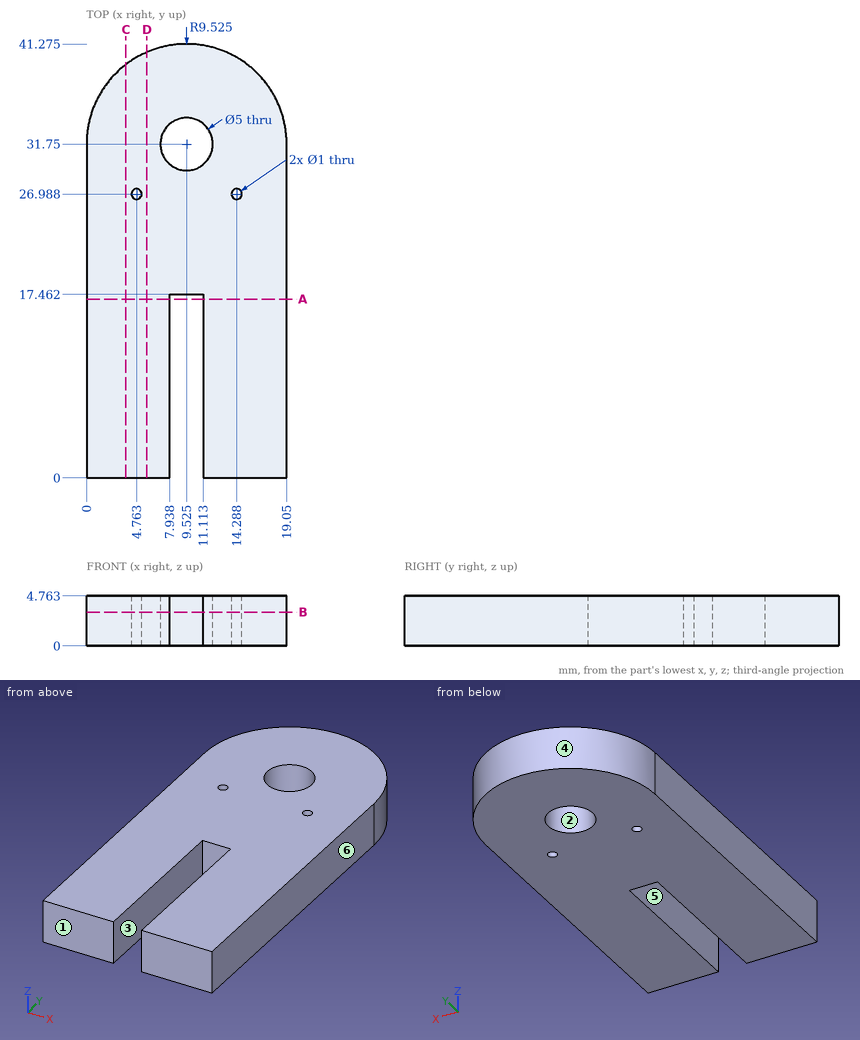
Print and shaded views of the part. All mm, measured from the part's lowest x, y and z. A direction names the side the tool comes from. Give positions to 0.01 mm unless a question says otherwise; leave off trailing zeros. Loops run counter-clockwise (first coordinate to the right, second up) from the corner with the lowest first, then second, coordinate; pieces in that order, holes last.
1) Pull direction X, two halves, no side cores. Call the marked faces 1, 2, 3 and 4: +X half, -X half, draft (parallel to the pull), parting line (faces both ways), or undercut.
2) Saw through at B-B (z = 3.2). Count the separate pieces of the cut face and the enclosed holes in it, plus the area to 3 significant figures.
3) Tool access for the marked faces 5 and 6: list every direction of +Z, -Z, +X, -X, +Y, -Y with a clear straight run to the whole face (end or side of a thin tool).
4) Flat gauge pins, fed straight in: pin 1 Ø8 at (x, y) = (7, 18.5) entering from -Z; pin 2 Ø1 at (x, z) = (9, 2.5) entering from -Y. Where does each tip first touch, or does it go through?
5) Saw through at D-D (x = 5.75). Write the cut outline in (y, z) (1 decimal), plus the area to 3 significant figures.
6) Saw through at A-A (y = 17). Write the cut outline in (x, z).
7) Wall check: line 1 (X direction, y = 10.5, z = 1.6); line 2 (X direction, y = 30, z = 4.2); line 3 (Y direction, x = 7.5, z = 0.2) (1 decimal). Give the ranges that are in metal, low to high.
8) Saw through at C-C (x = 3.75). Write the cut outline in (y, z) (1 decimal).
Answer block:
1. face 1: draft
1. face 2: undercut
1. face 3: undercut
1. face 4: parting line
2. separate pieces: 1
2. enclosed holes: 3
2. area: 671 mm2
3. face 5: +Z, -Z, -Y
3. face 6: +Z, -Z, +X, +Y, -Y
4. pin 1: stops at z = 0
4. pin 2: stops at y = 17.46
5. outline: (0, 0) - (40.5, 0) - (40.5, 4.8) - (0, 4.8) - close
5. area: 193 mm2
6. outline: (0, 0) - (7.94, 0) - (7.94, 4.76) - (0, 4.76) - close; (11.11, 0) - (19.05, 0) - (19.05, 4.76) - (11.11, 4.76) - close
7. line 1: x = 0 to 7.94, 11.11 to 19.05
7. line 2: x = 0 to 7.74, 11.31 to 19.05
7. line 3: y = 0 to 30.3, 33.2 to 41.1
8. outline: (0, 0) - (39.3, 0) - (39.3, 4.8) - (0, 4.8) - close
